```python
from build123d import *

# Parameters (mm, degrees)
SKETCH_3_W          = 27.8
SKETCH_3_H          = 15.9
EXTRUDE_1_DEPTH     = 10.3
SKETCH_4_R          = 1.55
CUT_EXTRUDE_1_DEPTH = 10.3
SKETCH_5_W          = 8
SKETCH_5_H          = 0.784988322
EXTRUDE_2_DEPTH     = 10.3
EXTRUDE_3_DEPTH     = 10.3


with BuildPart() as part:
    # 草图3 → 凸台-拉伸1 (new body)
    with BuildSketch(Plane.XY):
        with Locations((-13.9, 7.95)):
            Rectangle(SKETCH_3_W, SKETCH_3_H)
    extrude(amount=EXTRUDE_1_DEPTH)

    # 草图4 → 切除-拉伸1 (cut)
    with BuildSketch(Plane.XY.offset(10.3)):
        with Locations((-2.8, 13.1)):
            Circle(SKETCH_4_R)
        with Locations((-25, 2.8)):
            Circle(SKETCH_4_R)
    extrude(amount=-CUT_EXTRUDE_1_DEPTH, mode=Mode.SUBTRACT)

    # 草图5 → 凸台-拉伸2 (add)
    with BuildSketch(Plane.XY.offset(10.3)):
        with Locations((4, 10.95)):
            Rectangle(SKETCH_5_W, SKETCH_5_H)
        with Locations((4, 4.95)):
            Rectangle(SKETCH_5_W, SKETCH_5_H)
    extrude(amount=-EXTRUDE_2_DEPTH)

    # 草图6 → 凸台-拉伸3 (add)
    with BuildSketch(Plane.XY.offset(10.3)):
        with BuildLine():
            Line((-31.9, 18), (-22.452464215, 18))
            Line((-22.452464215, 18), (-10.9, 18))
            Line((-10.9, 18), (-10.9, 15.9))
            Line((-10.9, 15.9), (-11.6, 15.9))
            Line((-11.6, 15.9), (-11.6, 17.3))
            Line((-11.6, 17.3), (-31.896338759, 17.3))
            Line((-31.896338759, 17.3), (-32.6, 17.3))
            Line((-32.6, 17.3), (-32.6, 18))
            ThreePointArc((-32.6, 18), (-35.4, 20.8), (-38.2, 18))
            Line((-38.2, 18), (-38.9, 18))
            ThreePointArc((-38.9, 18), (-35.4, 21.5), (-31.9, 18))
        make_face()
    extrude(amount=-EXTRUDE_3_DEPTH)


solid = part.part
```
Geometry check sheet. Reference: the model listing, model coordinates, mm. A direction names the side the tool comes from. Give positions to 0.01 mm unless a question says otherwise; leave off trailing zeros. Order: outer loops, then holes, each group sorted by start corner. A loop starts at its lowest first (then second) coordinate and runs counter-clockwise, first axis right, second up.
1. Release check for a two-part mould opening along Y. For faces 5 (the face through (0, 8, 5)), 6 (the face through (-22, 18, 5)), 7 (the face through (-11, 9, 0)), 8 (the face through (-23.568, 2.206, 5.222)) record: pulls with the +Y half, pulls with the -Y half, needs draft (parallel to the pull), parting line crosses it, or undercut.
2. Section check A-A, the plane y = 2.8. Enter the section's corners in (x, z), and give its area (3 significant figures).
3. Thickness scan on L1, parallel to Y at x = 0.5, z = 10; L2, parallel to Y at x = -13.5, z = 1.5; L3, parallel to Y at x = -25.5, z = 4.25. Record the ranges inside material, lowest first.
4. Section check D-D, the plane x = -24. Enter the section's corners in (y, z), and give its area (3 significant figures).
5. Gauge pin test, flat ends, axial feed: pin 1 Ø6 at (x, z) = (-17, 3) entering from +Y; pin 2 Ø1.4 at (y, z) = (2, 4) entering from +X; pin 3 Ø2.5 at (y, z) = (17.5, 7) entering from +X; pin 4 Ø2.5 at (x, y) = (-2.8, 13.1) entering from -Z. Record the tip position at first contact, or that the pin passes through.
6. Section check C-C, the plane z = 8.75. Enter the section's corners in (x, y).
7. Section check B-B, the plane x = -2.8. Enter the section's corners in (y, z).
8. Access from +Z, -Z, +X, -X, +Y, -Y to the whole of each face (thin tool, end or side, straight path). Record for faces 1 (the face through (-22, 17.3, 5)), 2 (the face through (-6, 15.9, 5)), 3 (the face through (4, 10.558, 5)), 4 (the face through (4, 4.558, 5)).
Values follow:
1. face 5: undercut
1. face 6: pulls with the +Y half
1. face 7: needs draft
1. face 8: undercut
2. outline: (-27.8, 0) - (-26.55, 0) - (-26.55, 10.3) - (-27.8, 10.3) - close; (-23.45, 0) - (0, 0) - (0, 10.3) - (-23.45, 10.3) - close
2. area: 254 mm2
3. L1: y = 4.56 to 5.34, 10.56 to 11.34
3. L2: y = 0 to 15.9, 17.3 to 18
3. L3: y = 0 to 1.33, 4.27 to 15.9, 17.3 to 18
4. outline: (0, 0) - (1.62, 0) - (1.62, 10.3) - (0, 10.3) - close; (3.98, 0) - (15.9, 0) - (15.9, 10.3) - (3.98, 10.3) - close; (17.3, 0) - (18, 0) - (18, 10.3) - (17.3, 10.3) - close
4. area: 147 mm2
5. pin 1: stops at y = 18
5. pin 2: stops at x = 0
5. pin 3: stops at x = -10.9
5. pin 4: passes through
6. outline: (-38.9, 18) - (-38.2, 18) arc R2.8 cw to (-32.6, 18) - (-32.6, 17.3) - (-11.6, 17.3) - (-11.6, 15.9) - (-27.8, 15.9) - (-27.8, 0) - (0, 0) - (0, 4.56) - (8, 4.56) - (8, 5.34) - (0, 5.34) - (0, 10.56) - (8, 10.56) - (8, 11.34) - (0, 11.34) - (0, 15.9) - (-10.9, 15.9) - (-10.9, 18) - (-31.9, 18) arc R3.5 ccw to start; hole circle Ø3.1 at (-25, 2.8); hole circle Ø3.1 at (-2.8, 13.1)
7. outline: (0, 0) - (11.55, 0) - (11.55, 10.3) - (0, 10.3) - close; (14.65, 0) - (15.9, 0) - (15.9, 10.3) - (14.65, 10.3) - close
8. face 1: +Z, -Z, -X
8. face 2: +Z, -Z, +X, +Y
8. face 3: +Z, -Z, +X
8. face 4: +Z, -Z, +X, -Y
